Source: three-view drawing plus pictorial views. Frame: mm from the lowest corner of the part. A direction names the side the tool comes from. Round coordinates to 2 decimals unless told otherwise and drop trailing zeros. Loops run counter-clockwise (first coordinate to the right, second up) from the corner with the lowest first, then second, coordinate; pieces in that order, holes last. Notation, with made-up numbers: M -27,26.25 L -11,26.25 A6 cw -11,32.25 Z; hole C 65,-30.75 d11. An arc over 180 degrees is marked long. Answer as a JSON object with one key per item and string values.
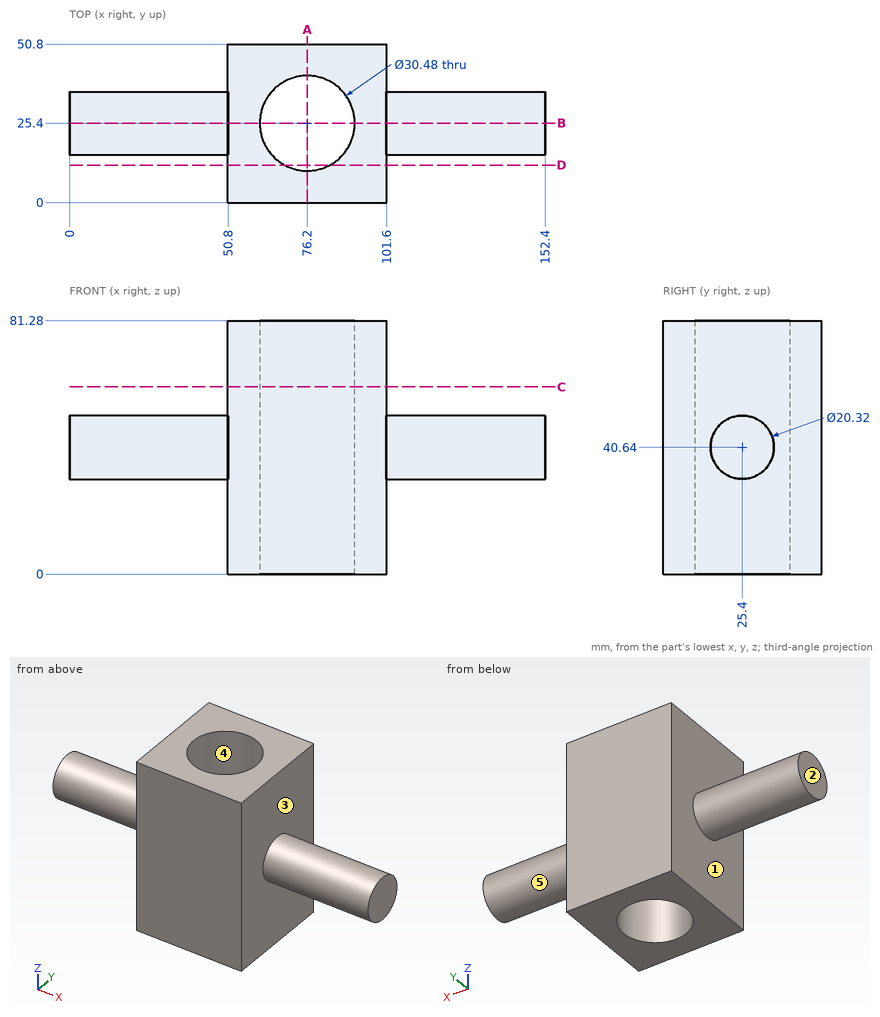
1) Line query: probe 1 along Y at (x, z) = (76.2, 39.5); probe 2 along X at (y, z) = (29.5, 18); probe 3 along X at (y, z) = (3.5, 12.5). Output: solid intervals per line, ascending.
Geometry results:
{"probe 1": "0 to 10.16, 40.64 to 50.8", "probe 2": "50.8 to 61.52, 90.88 to 101.6", "probe 3": "50.8 to 101.6"}
2) Cut plane D-D on y = 12. Return the cut outline in (x, z), and give its area (3 significant figures).
Geometry results:
{"outline": "M 50.8,0 L 68.94,0 L 68.94,81.28 L 50.8,81.28 Z; M 83.46,0 L 101.6,0 L 101.6,81.28 L 83.46,81.28 Z", "area": "2,950 mm2"}
3) Cut plane B-B on y = 25.4. Return the cut outline in (x, z), and give its area (3 significant figures).
Geometry results:
{"outline": "M 0,30.48 L 50.8,30.48 L 50.8,0 L 60.96,0 L 60.96,81.28 L 50.8,81.28 L 50.8,50.8 L 0,50.8 Z; M 91.44,0 L 101.6,0 L 101.6,30.48 L 152.4,30.48 L 152.4,50.8 L 101.6,50.8 L 101.6,81.28 L 91.44,81.28 Z", "area": "3,720 mm2"}
4) First-contact query: pin 1 (4 mm diameter, centred on x = 102, y = 18, fed in from +Z); pin 2 (2 mm diameter, centred on x = 129.5, y = 25.5, fed in from -Z); pin 3 (4 mm diameter, centred on y = 23, z = 73, fed in from -X); pin 4 (1 mm diameter, centred on y = 21.5, z = 56, fed in from +X). Flat tips, straight axial feed; report the tip coordinate or a pass-through.
Geometry results:
{"pin 1": "z = 81.28", "pin 2": "z = 30.48", "pin 3": "x = 50.8", "pin 4": "x = 101.6"}
5) Pull-direction query (X, two-part tool) for the marked faces 3, 4 and 5; classes: +X half, -X half, draft (parallel to the pull), parting line (faces both ways), or undercut.
Geometry results:
{"face 3": "+X half", "face 4": "undercut", "face 5": "draft"}
6) Set-up query: the marked faces 1 and 2. Return all of +Z, -Z, +X, -X, +Y, -Y with unobstructed straight access to the full face (end or side cutting, diameter ignored); none if empty.
Geometry results:
{"face 1": "-X", "face 2": "+Z, -Z, -X, +Y, -Y"}
7) Cut plane C-C on z = 60. Return the cut outline in (x, y).
Geometry results:
{"outline": "M 50.8,0 L 101.6,0 L 101.6,50.8 L 50.8,50.8 Z; hole C 76.2,25.4 d30.48"}
8) Cut plane A-A on x = 76.2. Return the cut outline in (y, z), and give its area (3 significant figures).
Geometry results:
{"outline": "M 0,0 L 10.16,0 L 10.16,81.28 L 0,81.28 Z; M 40.64,0 L 50.8,0 L 50.8,81.28 L 40.64,81.28 Z", "area": "1,650 mm2"}
